```python
from build123d import *

# Parameters (mm, degrees)
F0_W      = 51
F0_H      = 27
F1_DEPTH  = 7
F2_W      = 2.5
F2_H      = 13
F3_DEPTH  = 2.3
F5_DEPTH  = 51
F7_R      = 7.7
F8_DEPTH  = 46.5
F9_R      = 1.25
F10_DEPTH = 25
F11_R     = 2.35
F11_R_2   = 1.25
F12_DEPTH = 2
F13_R     = 2


with BuildPart() as f1:
    # F0 (on Front) → F1 (new body)
    with BuildSketch(Plane.XZ):
        with Locations((25.5, 13.5)):
            Rectangle(F0_W, F0_H)
    extrude(amount=F1_DEPTH)

    # F2 (on face) → F3 (join)
    with BuildSketch(Plane(origin=(0, 0, 0), x_dir=(-1, 0, 0), z_dir=(0, 1, 0))):
        with Locations((-49.75, 11.331)):
            Rectangle(F2_W, F2_H)
        with Locations((-1.25, 11.331)):
            Rectangle(F2_W, F2_H)
    extrude(amount=F3_DEPTH)

    # F4 (on face) → F5 (cut, through all)
    with BuildSketch(Plane.YZ.offset(51)):
        with BuildLine():
            Line((2.3, 7.1063698387), (2.3, 15.5556301613))
            ThreePointArc((2.3, 15.5556301613), (-0.65, 11.331), (2.3, 7.1063698387))
        make_face()
        with BuildLine():
            ThreePointArc((2.3, 7.1063698387), (6.4263346056, 7.6414878371), (8.35, 11.331))
            ThreePointArc((8.35, 11.331), (6.4263346056, 15.0205121629), (2.3, 15.5556301613))
            Line((2.3, 15.5556301613), (2.3, 7.1063698387))
        make_face()
    extrude(amount=-F5_DEPTH, mode=Mode.SUBTRACT)

    # F7 (on offset) → F8 (cut, through all)
    with BuildSketch(Plane.YZ.offset(49)):
        with Locations((3.85, 11.331)):
            Circle(F7_R)
    extrude(amount=-F8_DEPTH, mode=Mode.SUBTRACT)

    # F9 (on face) → F10 (cut)
    with BuildSketch(Plane(origin=(0, 0, 0), x_dir=(-1, 0, 0), z_dir=(0, 1, 0))):
        with Locations((-38.5, 23.25)):
            Circle(F9_R)
        with Locations((-12.5, 23.25)):
            Circle(F9_R)
    extrude(amount=-F10_DEPTH, mode=Mode.SUBTRACT)

    # F11 (on face) → F12 (cut)
    with BuildSketch(Plane.XZ.offset(7)):
        with Locations((12.5, 23.25)):
            Circle(F11_R)
        with Locations((12.5, 23.25)):
            Circle(F11_R_2, mode=Mode.SUBTRACT)
        with Locations((38.5, 23.25)):
            Circle(F11_R)
        with Locations((38.5, 23.25)):
            Circle(F11_R_2, mode=Mode.SUBTRACT)
    extrude(amount=-F12_DEPTH, mode=Mode.SUBTRACT)

    # F13
    f13_edges = [f1.edges().sort_by_distance(p)[0] for p in [
        (0, -3.5, 27),
        (51, -3.5, 27),
    ]]
    fillet(f13_edges, radius=F13_R)


solid = f1.part
```
CAD build for the part. Positions are in the model's coordinates, mm. A direction names the side the tool comes from. Round coordinates to 2 decimals unless told otherwise and drop trailing zeros. Order: outer loops, then holes, each group sorted by start corner. A loop starts at its lowest first (then second) coordinate and runs counter-clockwise, first axis right, second up.
Q1. Slice it at B-B (x = 12.5). Write the cut outline in (y, z), and give its area (3 significant figures).
Q2. Two-plate mould, pull along X, no slides. Class faces 1 (the flat face through (51, -3, 12)), 2 (the cylindrical face through (50.01, -0.65, 11.41)), 3 (the cylindrical face through (39.5, -2.5, 22.5)): pulls with the +X half, pulls with the -X half, needs draft (parallel to the pull), parting line crosses it, or undercut.
Q3. Slice it at C-C (y = 1.5). Write the cut outline in (x, z).
Q4. Drop flat-ended pins along their axis: pin 1 (0.7 mm diameter, centred on x = 2, y = 1, fed in from +Z); pin 2 (2.5 mm diameter, centred on x = 12, z = 23, fed in from -Y); pin 3 (7.5 mm diameter, centred on x = 15, z = 21, fed in from +Y). Give the stop position or say it passes through.
Q5. Slice it at A-A (z = 23.25). Write the cut outline in (x, y), and give its area (3 significant figures).
Q6. Slice it at D-D (x = 30.5). Write the cut outline in (y, z), and give its area (3 significant figures).
Q7. Wall check: L1, parallel to X at y = -1.5, z = 23.25; L2, parallel to Z at x = 12.5, y = -5.4; L3, parallel to X at y = -2, z = 11.5. Give the ranges that are in metal, low to high.
Q8. Which spindle directions (+Z, -Z, +X, -X, +Y, -Y) get a long thin tool onto all of the face, cutting with end or side? Do faces 4 (the flat face through (50, 1, 17.831)), 5 (the flat face through (1, 1, 4.831)), 6 (the cylindrical face through (39.584, -6.014, 21.165)). Say none if no direction does.
Results below:
1. outline: (-7, 0) - (0, 0) - (0, 4.66) arc R7.7 cw to (0, 18) - (0, 22) - (-5, 22) - (-5, 20.9) - (-7, 20.9) - close; (-7, 25.6) - (-5, 25.6) - (-5, 24.5) - (0, 24.5) - (0, 27) - (-7, 27) - close
1. area: 131 mm2
2. face 1: pulls with the +X half
2. face 2: needs draft
2. face 3: undercut
3. outline: (0, 4.83) - (2.5, 4.83) - (2.5, 7.49) - (0, 7.49) - close; (0, 15.17) - (2.5, 15.17) - (2.5, 17.83) - (0, 17.83) - close; (49, 4.83) - (51, 4.83) - (51, 7.49) - (49, 7.49) - close; (49, 15.17) - (51, 15.17) - (51, 17.83) - (49, 17.83) - close
4. pin 1: stops at z = 17.83
4. pin 2: stops at y = -5
4. pin 3: stops at y = 0
5. outline: (0, -7) - (10.15, -7) - (10.15, -5) - (11.25, -5) - (11.25, 0) - (0, 0) - close; (13.75, -5) - (14.85, -5) - (14.85, -7) - (36.15, -7) - (36.15, -5) - (37.25, -5) - (37.25, 0) - (13.75, 0) - close; (39.75, -5) - (40.85, -5) - (40.85, -7) - (51, -7) - (51, 0) - (39.75, 0) - close
5. area: 313 mm2
6. outline: (-7, 0) - (0, 0) - (0, 4.66) arc R7.7 cw to (0, 18) - (0, 27) - (-7, 27) - close
6. area: 153 mm2
7. L1: x = 0 to 11.25, 13.75 to 37.25, 39.75 to 51
7. L2: z = 0 to 20.9, 25.6 to 27
7. L3: x = 0 to 2.5, 49 to 51
8. face 4: +Z, +X, -X, +Y
8. face 5: -Z, +X, -X, +Y
8. face 6: -Y
